Verification items for the finished model (mm, model axes). A direction names the side the tool comes from. Round coordinates to 2 decimals unless told otherwise and drop trailing zeros. Write each loop counter-clockwise with the first axis right and the second up, starting at its lowest first coordinate (ties: lowest second). Pieces come first, ordered by that corner, then holes.
from build123d import *

# Parameters (mm, degrees)
ESQUISSE1_W             = 10
ESQUISSE1_H             = 50
BOSS_EXTRU_1_DEPTH      = 65
ENL_V_MAT_EXTRU_1_DEPTH = 110


with BuildPart() as part:
    # Esquisse1 → Boss.-Extru.1 (new body, symmetric)
    with BuildSketch(Plane.XY):
        Rectangle(ESQUISSE1_W, ESQUISSE1_H)
    extrude(amount=BOSS_EXTRU_1_DEPTH, both=True)

    # Esquisse2 → Enlèv. mat.-Extru.1 (cut)
    with BuildSketch(Plane(origin=(5, 0, 0), x_dir=(0, 0, -1), z_dir=(1, 0, 0))):
        with BuildLine():
            Line((-35, 10), (15, 10))
            ThreePointArc((15, 10), (25, 0), (15, -10))
            Line((15, -10), (-35, -10))
            ThreePointArc((-35, -10), (-45, 0), (-35, 10))
        make_face()
    extrude(amount=-ENL_V_MAT_EXTRU_1_DEPTH, mode=Mode.SUBTRACT)


solid = part.part
Q1. Tool access check on faces 1 (the cylindrical face through (0, 0, -25)), 2 (the flat face through (0, -25, 1)). Record the directions out of +Z, -Z, +X, -X, +Y, -Y that give a thin tool (end or side, any length) a straight path to the whole face; none if there is none.
Recorded:
face 1: +X, -X
face 2: +Z, -Z, +X, -X, -Y
Q2. Release check for a two-part mould opening along Z. For faces 3 (the flat face through (0, -10, 10)), 4 (the flat face through (0, 0, 65)), 5 (the flat face through (0, 25, 1)) record: released by +Z, released by -Z, zero draft, split by the parting line, or undercut.
Recorded:
face 3: undercut
face 4: released by +Z
face 5: zero draft
Q3. Sectioned sample at C-C (x = -3.5). Enter the section's corners in (y, z).
Recorded:
outline: (-25, -65) - (25, -65) - (25, 65) - (-25, 65) - close; hole (-10, -15) arc R10 ccw to (10, -15) - (10, 35) arc R10 ccw to (-10, 35) - close
Q4. Sectioned sample at B-B (z = 33.5). Enter the section's corners in (x, y).
Recorded:
outline: (-5, -25) - (5, -25) - (5, -10) - (-5, -10) - close; (-5, 10) - (5, 10) - (5, 25) - (-5, 25) - close
Q5. Sectioned sample at A-A (y = 0). Enter the section's corners in (x, z).
Recorded:
outline: (-5, -65) - (5, -65) - (5, -25) - (-5, -25) - close; (-5, 45) - (5, 45) - (5, 65) - (-5, 65) - close
Q6. Material ranges on line 1 along Y through (x, z) = (-0.5, 23); line 2 along Z through (x, y) = (-3.5, -0.5); line 3 along Z through (x, y) = (3, -5.5), recorded low to high.
Recorded:
line 1: y = -25 to -10, 10 to 25
line 2: z = -65 to -24.99, 44.99 to 65
line 3: z = -65 to -23.35, 43.35 to 65
